Input: part model. Units: mm. Frame: model coordinates. A direction names the side the tool comes from. Give positions to 0.01 mm unless a question says otherwise; leave off trailing zeros. Write each loop counter-clockwise with the first axis right and the second up, starting at its lowest first coordinate (ties: lowest second). Pieces come first, ordered by that corner, then holes. Notation, with made-up numbers: (70, -24) - (88, -24) arc R11 ccw to (88, -14) - close; hole circle Ø10 at (-13.5, 6). An arc over 180 degrees is marked (long way). Answer as CSV lines item,"result".
```python
from build123d import *

# Parameters (mm, degrees)
F2_DEPTH      = 31.75
F2_DEPTH_BACK = 31.75
F3_DEPTH      = 64.516
F3_DEPTH_BACK = 80.518
F4_R          = 4.7625
F5_DEPTH      = 25.4


with BuildPart() as f2:
    # F1 (on Front) → F2 (new body, two sides)
    with BuildSketch(Plane.XZ) as f2_sk:
        Polygon((47.625, 34.925), (15.875, 34.925), (15.875, 58.4651280605), (-3.175, 39.4151280605), (-3.175, 58.4651280605), (-22.225, 39.4151280605), (-22.225, 58.4651280605), (-47.625, 33.0651280605), (-47.625, -34.925), (47.625, -34.925), align=None)
    extrude(amount=F2_DEPTH)
    extrude(f2_sk.sketch, amount=-F2_DEPTH_BACK)

    # F0 (on Front) → F3 (cut, two sides)
    with BuildSketch(Plane.XZ) as f3_sk:
        Polygon((-44.45, -31.75), (44.45, -31.75), (44.45, 31.75), (12.7, 31.75), (12.7, 50.8), (-6.35, 31.75), (-6.35, 50.8), (-25.4, 31.75), (-25.4, 50.8), (-44.45, 31.75), align=None)
    extrude(amount=-F3_DEPTH, mode=Mode.SUBTRACT)
    extrude(f3_sk.sketch, amount=F3_DEPTH_BACK, mode=Mode.SUBTRACT)

    # F4 (on face) → F5 (join)
    with BuildSketch(Plane.XY.offset(34.925)):
        with Locations((31.75, 19.461568445)):
            Circle(F4_R)
        with Locations((31.75, 0.411568445)):
            Circle(F4_R)
        with Locations((31.75, -18.638431555)):
            Circle(F4_R)
    extrude(amount=F5_DEPTH)


solid = f2.part
```
Item 1: Cut plane C-C on y = 6.5. Return the cut outline in (x, z) (3 decimals), plus the area to 3 significant figures.
The answers:
outline,"(-47.625, -34.925) - (47.625, -34.925) - (47.625, 34.925) - (15.875, 34.925) - (15.875, 58.465) - (-3.175, 39.415) - (-3.175, 58.465) - (-22.225, 39.415) - (-22.225, 58.465) - (-47.625, 33.065) - close; hole (-44.45, -31.75) - (44.45, -31.75) - (44.45, 31.75) - (12.7, 31.75) - (12.7, 50.8) - (-6.35, 31.75) - (-6.35, 50.8) - (-25.4, 31.75) - (-25.4, 50.8) - (-44.45, 31.75) - close"
area,"1,270 mm²"
Item 2: Cut plane D-D on x = -36. Return the cut outline in (y, z) (3 decimals), plus the area to 3 significant figures.
The answers:
outline,"(-31.75, -34.925) - (31.75, -34.925) - (31.75, -31.75) - (-31.75, -31.75) - close; (-31.75, 40.2) - (31.75, 40.2) - (31.75, 44.69) - (-31.75, 44.69) - close"
area,"487 mm²"
Item 3: Cut plane A-A on x = 31.75. Return the cut outline in (y, z) (3 decimals).
The answers:
outline,"(-31.75, -34.925) - (31.75, -34.925) - (31.75, -31.75) - (-31.75, -31.75) - close; (-31.75, 31.75) - (31.75, 31.75) - (31.75, 34.925) - (24.224, 34.925) - (24.224, 60.325) - (14.699, 60.325) - (14.699, 34.925) - (5.174, 34.925) - (5.174, 60.325) - (-4.351, 60.325) - (-4.351, 34.925) - (-13.876, 34.925) - (-13.876, 60.325) - (-23.401, 60.325) - (-23.401, 34.925) - (-31.75, 34.925) - close"
Item 4: Ray query, line 1 (X direction, y = -12, z = 29) (3 decimals); line 2 (Z direction, x = 24, y = -2.5) (3 decimals); line 3 (X direction, y = -22.5, z = 32) (3 decimals). Return the intervals inside material, ascending. Write a range as from..to.
The answers:
line 1,"-47.625..-44.45, 44.45..47.625"
line 2,"-34.925..-31.75, 31.75..34.925"
line 3,"-47.625..-44.2, -25.4..-25.15, -6.35..-6.1, 12.7..47.625"
Item 5: Reachability of faces 3 (the face through (33.948, 15.236, 47.447)), 4 (the face through (-44.45, 0, 0)), 5 (the face through (-12.57, -0.44, 49.07)) from +Z, -Z, +X, -X, +Y, -Y: full face, straight path, thin tool, end or side. Return the list, or none.
The answers:
face 3,"+Z"
face 4,"+Y, -Y"
face 5,"+Z, +Y, -Y"
Item 6: Mould query, pull axis Y, two halves, no side actions, for faces 1 (the face through (15.875, 0, 47)), 2 (the face through (36.293, 1.842, 47.447)). Classes: +Y half, -Y half, draft (parallel to the pull), parting line (faces both ways), or undercut.
The answers:
face 1,"draft"
face 2,"undercut"
Item 7: Contact query for flat-ended pins moving along their axis: pin 1 (9.5 mm diameter, centred on y = -7, z = 50, fed in from +X); pin 2 (12 mm diameter, centred on y = -0.5, z = 46, fed in from +X); pin 3 (6 mm diameter, centred on x = -25.5, y = -11, fed in from +Z); pin 4 (8 mm diameter, centred on x = -18.5, z = 29, fed in from -Y). Output: stop coordinate, or through.
The answers:
pin 1,"x = 35.7"
pin 2,"x = 36.51"
pin 3,"z = 58.19"
pin 4,"through"
Item 8: Cut plane B-B on z = 0. Return the cut outline in (x, y) (3 decimals).
The answers:
outline,"(-47.625, -31.75) - (-44.45, -31.75) - (-44.45, 31.75) - (-47.625, 31.75) - close; (44.45, -31.75) - (47.625, -31.75) - (47.625, 31.75) - (44.45, 31.75) - close"
